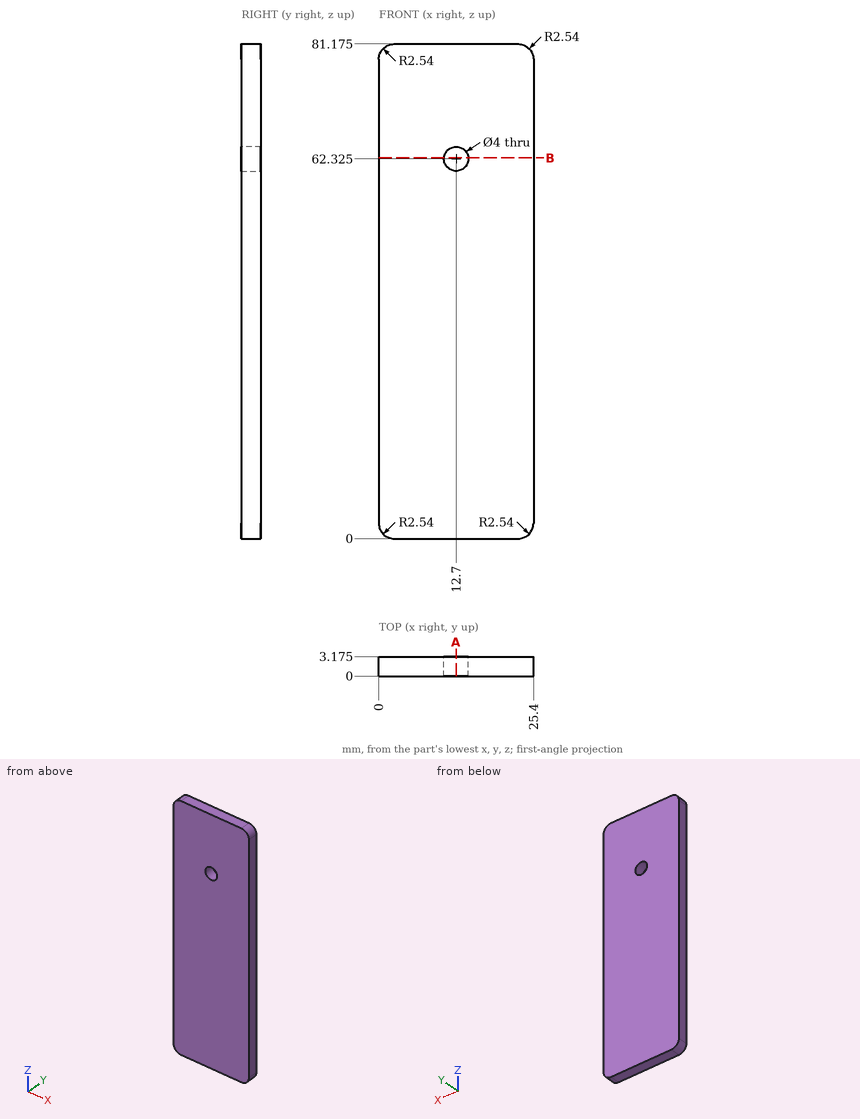
Print and shaded views of the part. All mm, measured from the part's lowest x, y and z. Give positions to 0.01 mm unless a question says otherwise; leave off trailing zeros. Write each loop counter-clockwise with the first axis right and the second up, starting at its lowest first coordinate (ties: lowest second). Pieces come first, ordered by that corner, then holes. Notation, with made-up numbers: M 5,30.25 L 39,30.25 A32 cw 39,62.25 Z; hole C 75.25,12.5 d11. An arc over 180 degrees is marked long. Use a Markdown table: item, result.
1) Cut at A-A (x = 12.7). List the corners of the cut face in (y, z) (3 decimals), and give its area (3 significant figures).
Responses:
| item | result |
|---|---|
| outline | M 0,0 L 3.175,0 L 3.175,60.325 L 0,60.325 Z; M 0,64.325 L 3.175,64.325 L 3.175,81.175 L 0,81.175 Z |
| area | 245 mm2 |
2) Pin check, flat tip, straight feed: pin 1 (1.5 mm diameter, centred on x = 17, z = 59, fed in from -Y). Stop position of the tip, or through.
Responses:
| item | result |
|---|---|
| pin 1 | stops at y = 0 |
3) Cut at B-B (z = 62.5). List the corners of the cut face in (x, y) (3 decimals).
Responses:
| item | result |
|---|---|
| outline | M 0,0 L 10.708,0 L 10.708,3.175 L 0,3.175 Z; M 14.692,0 L 25.4,0 L 25.4,3.175 L 14.692,3.175 Z |
4) Drill centre lines: line 1 (X direction, y = 0.3, z = 62.5); line 2 (Z direction, x = 12.75, y = 0.85) (3 decimals); line 3 (Z direction, x = 14.25, y = 0.2) (3 decimals). Where is each one in solid material? Low to high. Write a range as from..to.
Responses:
| item | result |
|---|---|
| line 1 | x = 0..10.71, 14.69..25.4 |
| line 2 | z = 0..60.326, 64.324..81.175 |
| line 3 | z = 0..61.061, 63.589..81.175 |
